For this review, take the finished solid that the model builds, in its own axes (mm). Face numbers are marked on the shaded views. Round coordinates to 2 decimals unless told otherwise and drop trailing zeros. Write each loop counter-clockwise with the first axis right and the second up, starting at its lowest first coordinate (ties: lowest second). Pieces come first, ordered by that corner, then holes.
from build123d import *

# Parameters (mm, degrees)
SKETCH2_W           = 100
SKETCH2_H           = 30
SKETCH2_R           = 11
BOSS_EXTRUDE1_DEPTH = 5
SKETCH3_W           = 5
SKETCH3_H           = 30
BOSS_EXTRUDE2_DEPTH = 25
SKETCH4_R           = 1
CUT_EXTRUDE1_DEPTH  = 106.475115549
SKETCH5_R           = 2
CUT_EXTRUDE2_DEPTH  = 10


with BuildPart() as part:
    # Sketch2 → Boss-Extrude1 (new body)
    with BuildSketch(Plane(origin=(0, 0, 0), x_dir=(1, 0, 0), z_dir=(0, 1, 0))):
        Rectangle(SKETCH2_W, SKETCH2_H)
        with Locations(Location((0, 0, 0), (0, 0, 270))):
            Circle(SKETCH2_R, mode=Mode.SUBTRACT)
    extrude(amount=BOSS_EXTRUDE1_DEPTH)

    # Sketch3 → Boss-Extrude2 (add)
    with BuildSketch(Plane(origin=(0, 5, 0), x_dir=(1, 0, 0), z_dir=(0, 1, 0))):
        with Locations((-47.5, 0)):
            Rectangle(SKETCH3_W, SKETCH3_H)
        with Locations((47.5, 0)):
            Rectangle(SKETCH3_W, SKETCH3_H)
    extrude(amount=BOSS_EXTRUDE2_DEPTH)

    # Sketch4 → Cut-Extrude1 (cut, through all)
    with BuildSketch(Plane(origin=(50, 0, 0), x_dir=(0, 0, -1), z_dir=(1, 0, 0))):
        with Locations((-7.5, 25)):
            Circle(SKETCH4_R)
        with Locations((7.5, 25)):
            Circle(SKETCH4_R)
    extrude(amount=-CUT_EXTRUDE1_DEPTH, mode=Mode.SUBTRACT)

    # Sketch5 → Cut-Extrude2 (cut)
    with BuildSketch(Plane.XZ):
        with Locations(Location((-22.5, -5, 0), (0, 0, 270))):
            Circle(SKETCH5_R)
        with Locations(Location((22.5, -5, 0), (0, 0, 270))):
            Circle(SKETCH5_R)
        with Locations(Location((-22.5, 5, 0), (0, 0, 270))):
            Circle(SKETCH5_R)
        with Locations(Location((22.5, 5, 0), (0, 0, 270))):
            Circle(SKETCH5_R)
    extrude(amount=-CUT_EXTRUDE2_DEPTH, mode=Mode.SUBTRACT)


solid = part.part
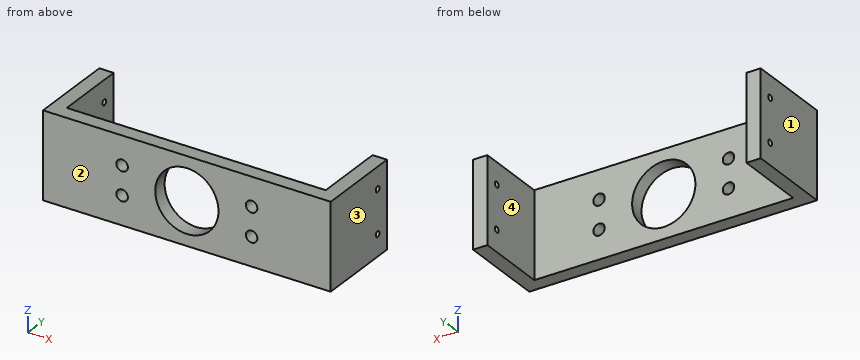
(1) We need section D-D, the plane x = -22.5. Give the boundary of the cut face in (y, z), and give its area (3 significant figures).
Geometry check:
outline: (0, -15) - (5, -15) - (5, -7) - (0, -7) - close; (0, -3) - (5, -3) - (5, 3) - (0, 3) - close; (0, 7) - (5, 7) - (5, 15) - (0, 15) - close
area: 110 mm2
(2) We need section A-A, the plane x = 0. Give the boundary of the cut face in (y, z).
Geometry check:
outline: (0, -15) - (5, -15) - (5, -11) - (0, -11) - close; (0, 11) - (5, 11) - (5, 15) - (0, 15) - close
(3) For line 1 along X through (y, z) = (15, 11); line 2 along X through (y, z) = (3.25, -5); line 3 along Y through (x, z) = (46.35, -7.5), list the stretches that pass through material, from the lowest coordinate up.
Geometry check:
line 1: x = -50 to -45, 45 to 50
line 2: x = -50 to -24.5, -20.5 to -9.8, 9.8 to 20.5, 24.5 to 50
line 3: y = 0 to 24, 26 to 30
(4) We need section C-C, the plane y = 23. Give the boundary of the cut face in (x, z), and give its area (3 significant figures).
Geometry check:
outline: (-50, -15) - (-45, -15) - (-45, 15) - (-50, 15) - close; (45, -15) - (50, -15) - (50, 15) - (45, 15) - close
area: 300 mm2
(5) For pin 1 Ø5 at (x, z) = (38, 8) entering from +Y; pin 2 Ø1.8 at (y, z) = (25, -7.5) entering from +X, all flat-tipped, find the tip position at first contact; note any pin that passes through.
Geometry check:
pin 1: stops at y = 5
pin 2: passes through
(6) We need section B-B, the plane z = 0. Give the boundary of the cut face in (x, y).
Geometry check:
outline: (-50, 0) - (-11, 0) - (-11, 5) - (-45, 5) - (-45, 30) - (-50, 30) - close; (11, 0) - (50, 0) - (50, 30) - (45, 30) - (45, 5) - (11, 5) - close
(7) Mouldability with a two-part tool opening along X and no side actions: class the marked faces 1, 2, 3 and 4 as pulls with the +X half, pulls with the -X half, needs draft (parallel to the pull), parting line crosses it, or undercut.
Geometry check:
face 1: pulls with the -X half
face 2: needs draft
face 3: pulls with the +X half
face 4: undercut
